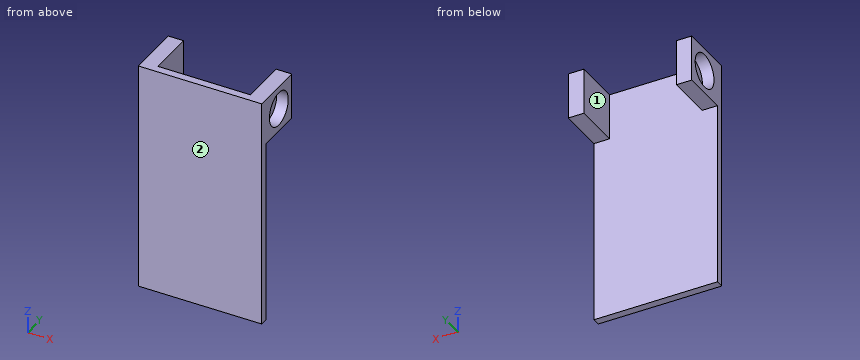
Autodesk Inventor part; units mm, degrees
ref_plane "YZ Plane" through (0, 0, 0) normal (1, 0, 0) x (0, 1, 0)
ref_plane "XZ Plane" through (0, 0, 0) normal (0, 1, 0) x (-1, 0, 0)
ref_plane "XY Plane" through (0, 0, 0) normal (0, 0, 1) x (1, 0, 0)
sketch "Sketch1" plane through (0, 0, 0) normal (0, 1, 0) x (-1, 0, 0)
  line L0 (-40, 50) -> (40, 50)
  line L1 (40, 50) -> (40, -50)
  line L2 (40, -50) -> (-40, -50)
  line L3 (-40, -50) -> (-40, 50)
  line L4 (-40, 50) -> (40, -50) construction
  line L5 (40, 50) -> (-40, -50) construction
  point P0 (0, 0)
  dimension "d0" = 80
  dimension "d1" = 100
extrude "Extrusion1" add sketch "Sketch1" along normal blind 5
sketch "Sketch2" plane through (0, 5, 0) normal (0, 1, 0) x (1, 0, 0)
  line L0 (-40, -50) -> (-30, -50)
  line L1 (-30, -50) -> (-30, -20)
  line L2 (-30, -20) -> (-40, -20)
  line L3 (-40, -20) -> (-40, -50)
  line L4 (40, -50) -> (30, -50)
  line L5 (30, -50) -> (30, -20)
  line L6 (30, -20) -> (40, -20)
  line L7 (40, -20) -> (40, -50)
  point P0 (0, 0)
  dimension "d4" = 10
  dimension "d5" = 30
  dimension "d6" = 10
  dimension "d7" = 30
extrude "Extrusion2" add sketch "Sketch2" along normal blind 30
sketch "Sketch3" plane through (-40, 0, -50) normal (-1, 0, 0) x (0, 0, 1)
  circle A0 centre (85, 20) radius 11
  point P0 (50, 0)
  dimension "d10" = 22
extrude "Extrusion3" cut sketch "Sketch3" against normal blind 7.5
sketch "Sketch4" plane through (40, 0, 50) normal (1, 0, 0) x (0, 0, -1)
  circle A0 centre (15, 20) radius 11
  circle A1 centre (15, 20) radius 11
  point P0 (50, 0)
extrude "Extrusion4" cut sketch "Sketch4" against normal blind 7.5
sketch "Sketch6" plane through (40, 0, -50) normal (0, 0, -1) x (-1, 0, 0)
  line L0 (80, 5) -> (0, 5)
  line L1 (0, 5) -> (0, 0)
  line L2 (0, 0) -> (80, 0)
  line L3 (80, 0) -> (80, 5)
  point P0 (40, 0)
extrude "Extrusion5" add sketch "Sketch6" along normal blind 50
properties part number "BassGtrBotBase"
Geometry: final body of the model. Coordinates: model frame, mm. Face numbers are marked on the shaded views. Give positions to 0.01 mm unless a question says otherwise; leave off trailing zeros. Loops run counter-clockwise (first coordinate to the right, second up) from the corner with the lowest first, then second, coordinate; pieces in that order, holes last. Notation, with made-up numbers: M 53,1.5 L 99,1.5 A12 ccw 99,15.5 Z; hole C 9,31.5 d2. An arc over 180 degrees is marked long. Put each result on its own line as item: value. Start each with the question number.
1) Pull-direction query (X, two-part tool) for the marked faces 1 and 2; classes: pulls with the +X half, pulls with the -X half, needs draft (parallel to the pull), parting line crosses it, or undercut.
2) Cut plane B-B (z = 35). Output: boundary loops of the cut face in (x, y), then the cut area to 3 significant figures.
3) Ray query, line 1 along X through (y, z) = (15, 33); line 2 along Y through (x, z) = (-35, 35); line 3 along X through (y, z) = (29, 20.5). Return the intervals inside material, ascending.
4) Contact query for flat-ended pins moving along their axis: pin 1 (12 mm diameter, centred on x = -19, z = -78.5, fed in from +Y); pin 2 (5 mm diameter, centred on x = 37, y = 19, fed in from -Z); pin 3 (5 mm diameter, centred on x = -27, y = 10.5, fed in from +Z); pin 4 (17.5 mm diameter, centred on y = 20, z = 35, fed in from +X). Output: stop coordinate, or through.
5) Cut plane D-D (z = 11). Output: boundary loops of the cut face in (x, y), then the cut area to 3 significant figures.
6) Cut plane A-A (y = 20). Output: boundary loops of the cut face in (x, z), then the cut area to 3 significant figures.
7) Cut plane C-C (x = -26). Output: boundary loops of the cut face in (y, z).
Verdict:
1. face 1: undercut
1. face 2: needs draft
2. outline: M -40,0 L 40,0 L 40,9 L 32.5,9 L 32.5,31 L 40,31 L 40,35 L 30,35 L 30,5 L -30,5 L -30,35 L -40,35 L -40,31 L -32.5,31 L -32.5,9 L -40,9 Z
2. area: 670 mm2
3. line 1: -32.5 to -30, 30 to 32.5
3. line 2: 0 to 9, 31 to 35
3. line 3: -40 to -30, 30 to 40
4. pin 1: y = 5
4. pin 2: z = 20
4. pin 3: through
4. pin 4: x = 32.5
5. outline: M -40,0 L 40,0 L 40,5 L -40,5 Z
5. area: 400 mm2
6. outline: M -40,20 L -30,20 L -30,50 L -40,50 L -40,46 L -32.5,46 L -32.5,24 L -40,24 Z; M 30,20 L 40,20 L 40,24 L 32.5,24 L 32.5,46 L 40,46 L 40,50 L 30,50 Z
6. area: 270 mm2
7. outline: M 0,-100 L 5,-100 L 5,50 L 0,50 Z
